Geometry: final body of the model. Coordinates: model frame, mm. A direction names the side the tool comes from. Give positions to 0.01 mm unless a question says otherwise; leave off trailing zeros. Loops run counter-clockwise (first coordinate to the right, second up) from the corner with the lowest first, then second, coordinate; pieces in that order, holes last. Notation, with made-up numbers: M 83.25,6 L 123.25,6 A5 cw 123.25,12 Z; hole C -1.5,14.25 d8. An arc over 180 degrees is marked long. Put each result on its own line as item: value.
```python
from build123d import *

# Parameters (mm, degrees)
F0_W     = 1000
F0_H     = 1000
F0_W_2   = 100
F0_H_2   = 100
F1_DEPTH = 100
F2_R     = 50
F4_DEPTH = 20
F5_W     = 50
F5_H     = 50
F6_DEPTH = 1000
F7_SIZE  = 10


with BuildPart() as f1:
    # F0 (on Top) → F1 (new body)
    with BuildSketch(Plane.XY):
        Rectangle(F0_W, F0_H)
        Polygon((62.132034, 150), (150, 62.132034), (150, -62.132034), (62.132034, -150), (-62.132034, -150), (-150, -62.132034), (-150, 62.132034), (-62.132034, 150), align=None, mode=Mode.SUBTRACT)
        with Locations((350, 350)):
            Rectangle(F0_W_2, F0_H_2, mode=Mode.SUBTRACT)
    extrude(amount=F1_DEPTH)

    # F2
    f2_edges = [f1.edges().sort_by_distance(p)[0] for p in [
        (0, -500, 100),
        (-500, 0, 100),
        (0, 500, 100),
        (500, 0, 100),
    ]]
    fillet(f2_edges, radius=F2_R)

    # F3 (on face) → F4 (join)
    with BuildSketch(Plane(origin=(0, 0, 0), x_dir=(1, 0, 0), z_dir=(0, 0, -1))):
        Polygon((150, -62.132034), (150, 62.132034), (62.132034, 150), (-62.132034, 150), (-150, 62.132034), (-150, -62.132034), (-62.132034, -150), (62.132034, -150), align=None)
    extrude(amount=-F4_DEPTH)

    # F5 (on face) → F6 (join)
    with BuildSketch(Plane(origin=(0, 0, 0), x_dir=(1, 0, 0), z_dir=(0, 0, -1))):
        with Locations((-465, 465)):
            Rectangle(F5_W, F5_H)
        with Locations((-465, -465)):
            Rectangle(F5_W, F5_H)
        with Locations((465, -465)):
            Rectangle(F5_W, F5_H)
        with Locations((465, 465)):
            Rectangle(F5_W, F5_H)
    extrude(amount=F6_DEPTH)

    # F7
    f7_edges = [f1.edges().sort_by_distance(p)[0] for p in [
        (150, 0, 20),
        (106.066017, -106.066017, 20),
        (0, -150, 20),
        (-106.066017, -106.066017, 20),
        (-150, 0, 20),
        (-106.066017, 106.066017, 20),
        (0, 150, 20),
        (106.066017, 106.066017, 20),
    ]]
    chamfer(f7_edges, length=F7_SIZE)


solid = f1.part
```
Item 1: Mould query, pull axis X, two halves, no side actions, for faces 1 (the flat face through (-465, 465, -1000)), 2 (the cylindrical face through (485.742, 7, 84.964)), 3 (the flat face through (-106.68, 105.45, 64.51)). Classes: pulls with the +X half, pulls with the -X half, needs draft (parallel to the pull), parting line crosses it, or undercut.
Output values:
face 1: needs draft
face 2: pulls with the +X half
face 3: undercut
Item 2: Section B-B on x = 378. Output: boundary loops of the cut face in (y, z).
Output values:
outline: M -500,0 L 300,0 L 300,100 L -450,100 A50 ccw -500,50 Z; M 400,0 L 500,0 L 500,50 A50 ccw 450,100 L 400,100 Z
Item 3: Line query: probe 1 along X at (y, z) = (-459.5, -946.5); probe 2 along Z at (x, y) = (-32.5, 121.5); probe 3 along Z at (x, y) = (449, 220). Output: solid intervals per line, ascending. Write a range as [from, to].
Output values:
probe 1: [-490, -440], [440, 490]
probe 2: [0, 20]
probe 3: [0, 100]
Item 4: Section C-C on x = 3. Output: boundary loops of the cut face in (y, z).
Output values:
outline: M -500,0 L 500,0 L 500,50 A50 ccw 450,100 L 150,100 L 150,30 L 140,20 L -140,20 L -150,30 L -150,100 L -450,100 A50 ccw -500,50 Z
Item 5: Set-up query: faces 4 (the flat face through (-465, -490, -493)), 5 (the flat face through (103.096, -101.866, 24.93)), 6 (the flat face through (349, 400, 49)). Return all of +Z, -Z, +X, -X, +Y, -Y with unobstructed straight access to the full face (end or side cutting, diameter ignored); none if empty.
Output values:
face 4: -Z, +X, -X, -Y
face 5: +Z
face 6: +Z, -Z
Item 6: Pin query (flat end, axial travel): pin 1 Ø15 at (x, z) = (-464, -737.5) entering from +Y; pin 2 Ø25 at (y, z) = (-472.5, -728) entering from -X; pin 3 Ø25 at (y, z) = (-472.5, -624) entering from +X. Return the tip coordinate at first contact, or that it passes through.
Output values:
pin 1: y = 490
pin 2: x = -490
pin 3: x = 490
Item 7: Section A-A on z = -218. Output: boundary loops of the cut face in (x, y), then the cut area to 3 significant figures.
Output values:
outline: M -490,-490 L -440,-490 L -440,-440 L -490,-440 Z; M -490,440 L -440,440 L -440,490 L -490,490 Z; M 440,-490 L 490,-490 L 490,-440 L 440,-440 Z; M 440,440 L 490,440 L 490,490 L 440,490 Z
area: 10,000 mm²
